Autodesk Inventor part; units mm, degrees
ref_plane "YZ Plane" through (0, 0, 0) normal (1, 0, 0) x (0, 1, 0)
ref_plane "XZ Plane" through (0, 0, 0) normal (0, 1, 0) x (-1, 0, 0)
ref_plane "XY Plane" through (0, 0, 0) normal (0, 0, 1) x (1, 0, 0)
sketch "Skizze1" plane through (0, 0, 0) normal (1, 0, 0) x (0, 1, 0)
  line L0 (0, 38.36) -> (0, -55.16)
  line L1 (-2, 0) -> (12, 0) construction
  line L2 (6, 0) -> (6, 25)
  line L3 (6, 25) -> (0, 25)
  line L4 (6, 0) -> (10, 0)
  line L5 (10, 0) -> (10, -21.8)
  line L6 (10, -21.8) -> (4, -21.8)
  line L7 (4, -21.8) -> (4, -41.8)
  line L8 (4, -41.8) -> (0, -41.8)
  line L9 (0, -41.8) -> (0, 25)
  point P0 (0, 0)
  dimension "d0" = 12
  dimension "d1" = 25
  dimension "d3" = 8
  dimension "d4" = 21.8
  dimension "d6" = 20
  dimension "d23" = 20
revolve "Grundkörper" add sketch "Skizze1" angle 360 about axis through (0, 0, 0) along (0, 0, -1)
thread "M8"
sketch "Skizze2" plane through (0, 0, 25) normal (0, 0, 1) x (1, 0, 0)
  circle A0 centre (0, 0) radius 6
hole "M5x10" at (0, 0, 25) direction (0, 0, -1) diameter 4.134 depth 14.2 tip angle 118 countersink diameter 5 countersink angle 90
sketch "Skizze3" plane through (0, 0, 0) normal (0, 1, 0) x (-1, 0, 0)
  line L0 (0, -24.96) -> (0, 4.16) construction
  line L1 (-10, -21.8) -> (10, -21.8) construction
  line L2 (10, 0) -> (10, -21.8) construction
  line L3 (-10, 0) -> (-10, -21.8) construction
  line L4 (8.5, -21.8) -> (8.5, -11.8)
  line L5 (8.5, -11.8) -> (10, -11.8)
  line L6 (10, -11.8) -> (10, -21.8)
  line L7 (10, -21.8) -> (8.5, -21.8)
  line L8 (-10, -11.8) -> (-8.5, -11.8)
  line L9 (-8.5, -11.8) -> (-8.5, -21.8)
  line L10 (-8.5, -21.8) -> (-10, -21.8)
  line L11 (-10, -21.8) -> (-10, -11.8)
  point P0 (0, 0)
  dimension "d24" = 10
  dimension "d25" = 17
extrude "Extrusion1" cut sketch "Skizze3" along normal through all both and the other way through all
properties part number "200-60-DIFFERENTIAL-CONNECTOR-02" material "Edelstahl"
The model under review builds one solid part; all positions refer to its coordinate system, in mm. A direction names the side the tool comes from. Give positions to 0.01 mm unless a question says otherwise; leave off trailing zeros. Order: outer loops, then holes, each group sorted by start corner. A loop starts at its lowest first (then second) coordinate and runs counter-clockwise, first axis right, second up. Notation, with made-up numbers: M 80,-23.5 L 132,-23.5 A27 cw 132,4.5 Z; hole C 33.5,57.25 d10. An arc over 180 degrees is marked long. Use one line per item in the form item = value. Start each with the question number.
Item 1: We need section A-A on z = 14. Give the boundary of the cut face in (x, y).
Item 2: We need section C-C on x = -4.75. Give the boundary of the cut face in (y, z), plus the area to 3 significant figures.
Item 3: We need section D-D on z = -10.5. Give the boundary of the cut face in (x, y), plus the area to 3 significant figures.
Item 4: We need section B-B on z = -25. Give the boundary of the cut face in (x, y), plus the area to 3 significant figures.
Item 5: The part is to be moulded in two halves that separate along X. For faces 5 (the flat face through (-4, 2, -21.8)), 6 (the cylindrical face through (1.26, 1.64, 17.59)), 7 (the conical face through (-0.137, -0.332, 9.774)), 8 (the flat face through (-8.5, 0, -17)), say which applies: pulls with the +X half, pulls with the -X half, needs draft (parallel to the pull), parting line crosses it, or undercut.
Item 6: To check wall thickness, follow line 1 along X through (y, z) = (0, 19.75); line 2 along Z through (x, y) = (-8.25, -3.5); line 3 along X through (y, z) = (5.25, -2). State the ranges of each line that lie inside material, in increasing order. Write a range as from..to.
Item 7: For faces 1 (the cylindrical face through (-3.905, -0.867, -31.94)), 2 (the flat face through (0, 7, 0)), 3 (the flat face through (8.5, 0, -17)), 4 (the flat face through (-9, 0, -11.8)), list the 3-axis set-ups (+Z, -Z, +X, -X, +Y, -Y) from which the entire face can be reached by the end or side of a thin tool; tool diameter is ignored.
Item 8: Insertion check: pin 1 Ø12 at (y, z) = (-3, -21) entering from +X; pin 2 Ø8 at (y, z) = (7, -21) entering from -X; pin 3 Ø1.5 at (y, z) = (-8, 13.5) entering from +X; pin 4 Ø0.5 at (x, y) = (9, 1.5) entering from -Z. Each pin has a flat end and moves straight along its axis. Give the tip position at first contact, or say it passes through.
Completed:
q1.outline = C 0,0 d12; hole C 0,0 d4.13
q2.outline = M -8.8,-21.8 L 8.8,-21.8 L 8.8,0 L 3.67,0 L 3.67,25 L -3.67,25 L -3.67,0 L -8.8,0 Z
q2.area = 567 mm²
q3.outline = C 0,0 d20
q3.area = 314 mm²
q4.outline = C 0,0 d8
q4.area = 50.3 mm²
q5.face_5 = needs draft
q5.face_6 = undercut
q5.face_7 = undercut
q5.face_8 = pulls with the -X half
q6.line_1 = -6..-2.07, 2.07..6
q6.line_2 = -21.8..0
q6.line_3 = -8.51..8.51
q7.face_1 = -Z
q7.face_2 = +Z
q7.face_3 = -Z, +X, +Y, -Y
q7.face_4 = -Z, -X, +Y, -Y
q8.pin_1 = 8.5
q8.pin_2 = -8.5
q8.pin_3 = through
q8.pin_4 = -11.8
